from build123d import *

# Parameters (mm, degrees)
CHAMFER1_SIZE = 1.7
FILLET4_R     = 2.6
FILLET7_R     = 2.6
FILLET8_R     = 2.6
FILLET9_R     = 2.6


with BuildPart() as part:
    # Sketch1 → Revolve3 (revolve)
    with BuildSketch(Plane.XY):
        Polygon((-22.55, 98.726264023), (-0.15, 98.726264023), (-0.15, -215.073735977), (-22.55, -215.073735977), (-22.55, -182.273735977), (-25.15, -182.273735977), (-25.15, -168.473735977), (-22.55, -168.473735977), (-22.55, -165.073735977), (-30.3, -165.073735977), (-30.3, 34.926264023), (-22.55, 34.926264023), (-22.55, 38.326264023), (-25.15, 38.326264023), (-25.15, 52.126264023), (-22.55, 52.126264023), align=None)
    revolve(axis=Axis((-0.15, 98.726264023, 0), (0, -1, 0)))

    # Chamfer1
    chamfer1_edges = [part.edges().sort_by_distance(p)[0] for p in [
        (22.25, 98.726264023, 0),
    ]]
    chamfer(chamfer1_edges, length=CHAMFER1_SIZE)

    # Fillet4
    fillet4_edges = [part.edges().sort_by_distance(p)[0] for p in [
        (22.25, 52.126264023, 0),
    ]]
    fillet(fillet4_edges, radius=FILLET4_R - 0.0001)  # a hair under: the kernel refuses the full size

    # Fillet7
    fillet7_edges = [part.edges().sort_by_distance(p)[0] for p in [
        (22.25, 38.326264023, 0),
    ]]
    fillet(fillet7_edges, radius=FILLET7_R - 0.0001)  # a hair under: the kernel refuses the full size

    # Fillet8
    fillet8_edges = [part.edges().sort_by_distance(p)[0] for p in [
        (22.25, -182.273735977, 0),
    ]]
    fillet(fillet8_edges, radius=FILLET8_R - 0.0001)  # a hair under: the kernel refuses the full size

    # Fillet9
    fillet9_edges = [part.edges().sort_by_distance(p)[0] for p in [
        (22.25, -168.473735977, 0),
    ]]
    fillet(fillet9_edges, radius=FILLET9_R - 0.0001)  # a hair under: the kernel refuses the full size


solid = part.part
Can you work these out from the model? Positions are in its coordinate system, mm. A direction names the side the tool comes from. Give positions to 0.01 mm unless a question says otherwise; leave off trailing zeros. Order: outer loops, then holes, each group sorted by start corner. A loop starts at its lowest first (then second) coordinate and runs counter-clockwise, first axis right, second up. Notation, with made-up numbers: M 77,28.25 L 81,28.25 A18 ccw 81,39.25 Z; hole C 0.25,55 d10. An arc over 180 degrees is marked long. Use a Markdown table: item, result. Add a question column.
Item 1: We'd pull the mould along Y, two halves only. Please class faces 1 (the conical face through (2.56, 98.62, -20.63)), 2 (the cylindrical face through (22.23, -165.47, -0.98)), 3 (the cylindrical face through (-24, 45.3, -7.5)): +Y half, -Y half, draft (parallel to the pull), parting line (faces both ways), or undercut.
Item 2: Will these pins go through, and if not, where does the flat tip stop? pin 1 (1.5 mm diameter, centred on y = -174.5, z = -14, fed in from +X); pin 2 (10 mm diameter, centred on y = -30, z = -11.5, fed in from +X); pin 3 (12 mm diameter, centred on x = -19.5, y = -20, fed in from +Z).
Item 3: For faces 4 (the flat face through (22.32, 34.926, 2.09)), 5 (the cylindrical face through (22.23, -199.76, -0.98)), 6 (the cylindrical face through (22.23, 76.17, -0.98)), which set-ups out of +Z, -Z, +X, -X, +Y, -Y let a thin tool reach every point of the face, with its end or its side?
Item 4: If I drill on L1, parallel to Y at x = 20, z = -13.5; L2, parallel to Y at x = -17, z = 17; L3, parallel to Y at x = -5.5, z = -20, over which ranges is the centre line in solid material (lowest first)? Write a range as [from, to].
Item 5: Suppose I cut it at A-A (y = -149.5). List the corners of the cut face in (x, z) for me.
Answer sheet:
| question | item | result |
|---|---|---|
| 1 | face 1 | +Y half |
| 1 | face 2 | undercut |
| 1 | face 3 | draft |
| 2 | pin 1 | stops at x = 21.05 |
| 2 | pin 2 | stops at x = 29.29 |
| 2 | pin 3 | stops at z = 27.03 |
| 3 | face 4 | none |
| 3 | face 5 | -Y |
| 3 | face 6 | +Y |
| 4 | L1 | y = [-182.38, -168.36], [-165.07, 34.93], [38.22, 52.24] |
| 4 | L2 | y = [-182.5, -168.25], [-165.07, 34.93], [38.1, 52.35] |
| 4 | L3 | y = [-215.07, 98.72] |
| 5 | outline | C -0.15,0 d60.3 |
